Autodesk Inventor part; units mm, degrees
ref_plane "YZ Plane" through (0, 0, 0) normal (1, 0, 0) x (0, 1, 0)
ref_plane "XZ Plane" through (0, 0, 0) normal (0, 1, 0) x (-1, 0, 0)
ref_plane "XY Plane" through (0, 0, 0) normal (0, 0, 1) x (1, 0, 0)
sketch "Sketch1" plane through (0, 0, 0) normal (0, 0, 1) x (1, 0, 0)
  line L0 (50, 829.4999) -> (50, 329.4999)
  line L1 (50, 329.4999) -> (-50, 329.4999)
  line L2 (-50, 329.4999) -> (-50, 829.4999)
  line L3 (-50, 829.4999) -> (-50, 887.2349)
  line L4 (-50, 829.4999) -> (7.735, 829.4999) construction
  line L5 (-50, 887.2349) -> (50, 829.4999)
  dimension "d2" = 57.735
  dimension "d3" = 90
  dimension "d6" = 500
  dimension "d7" = 500
extrude "Extrusion1" add sketch "Sketch1" along normal blind 20
Model file for the job. Use its own axes, mm. Give positions to 0.01 mm unless a question says otherwise; leave off trailing zeros. Order: outer loops, then holes, each group sorted by start corner. A loop starts at its lowest first (then second) coordinate and runs counter-clockwise, first axis right, second up.
1) Saw through at A-A, the plane z = 9. Write the cut outline in (x, y).
2) Pin check, flat tip, straight feed: pin 1 (4 mm diameter, centred on x = 0, z = 7, fed in from +Y). Stop position of the tip, or through.
3) Wall check: probe 1 along Y at (x, z) = (-19.5, 5.75); probe 2 along Y at (x, z) = (16, 16.25). Give the ranges that are in metal, low to high.
4) Saw through at B-B, the plane x = -30. Write the cut outline in (y, z).
Computed:
1. outline: (-50, 329.5) - (50, 329.5) - (50, 829.5) - (-50, 887.23) - close
2. pin 1: stops at y = 859.52
3. probe 1: y = 329.5 to 869.63
3. probe 2: y = 329.5 to 849.13
4. outline: (329.5, 0) - (875.69, 0) - (875.69, 20) - (329.5, 20) - close
